```python
from build123d import *

# Parameters (mm, degrees)
BOSS_EXTRUDE1_DEPTH = 600
SKETCH2_W           = 40
SKETCH2_H           = 20
BOSS_EXTRUDE2_DEPTH = 40
FILLET1_R           = 10
SKETCH3_R           = 12
CUT_EXTRUDE1_DEPTH  = 40


with BuildPart() as part:
    # Sketch1 → Boss-Extrude1 (new body)
    with BuildSketch(Plane(origin=(0, 0, 0), x_dir=(1, 0, 0), z_dir=(0, 1, 0))):
        with BuildLine():
            Line((9.494919477, 2.658080263), (9.010919477, 2.658080263))
            ThreePointArc((9.010919477, 2.658080263), (8.651709233, 2.806870018), (8.502919477, 3.166080263))
            Line((8.502919477, 3.166080263), (8.502919477, 5.515080263))
            ThreePointArc((8.502919477, 5.515080263), (8.354129722, 5.874290508), (7.994919477, 6.023080263))
            Line((7.994919477, 6.023080263), (7.269000139, 6.023080263))
            ThreePointArc((7.269000139, 6.023080263), (7.074596955, 5.984411065), (6.909789894, 5.874290508))
            Line((6.909789894, 5.874290508), (3.806709233, 2.771209846))
            ThreePointArc((3.806709233, 2.771209846), (3.696588675, 2.606402785), (3.657919477, 2.411999602))
            Line((3.657919477, 2.411999602), (3.657919477, -2.355839076))
            ThreePointArc((3.657919477, -2.355839076), (3.696588675, -2.550242259), (3.806709233, -2.71504932))
            Line((3.806709233, -2.71504932), (6.909789894, -5.818129982))
            ThreePointArc((6.909789894, -5.818129982), (7.074596955, -5.92825054), (7.269000139, -5.966919737))
            Line((7.269000139, -5.966919737), (7.994919477, -5.966919737))
            ThreePointArc((7.994919477, -5.966919737), (8.354129722, -5.818129982), (8.502919477, -5.458919737))
            Line((8.502919477, -5.458919737), (8.502919477, -3.109919737))
            ThreePointArc((8.502919477, -3.109919737), (8.651709233, -2.750709492), (9.010919477, -2.601919737))
            Line((9.010919477, -2.601919737), (9.494919477, -2.601919737))
            ThreePointArc((9.494919477, -2.601919737), (9.854129722, -2.750709492), (10.002919477, -3.109919737))
            Line((10.002919477, -3.109919737), (10.002919477, -8.471919737))
            ThreePointArc((10.002919477, -8.471919737), (9.563579649, -9.532579909), (8.502919477, -9.971919737))
            Line((8.502919477, -9.971919737), (3.140919477, -9.971919737))
            ThreePointArc((3.140919477, -9.971919737), (2.781709233, -9.823129982), (2.632919477, -9.463919737))
            Line((2.632919477, -9.463919737), (2.632919477, -8.979919737))
            ThreePointArc((2.632919477, -8.979919737), (2.781709233, -8.620709492), (3.140919477, -8.471919737))
            Line((3.140919477, -8.471919737), (5.489919477, -8.471919737))
            ThreePointArc((5.489919477, -8.471919737), (5.849129722, -8.323129982), (5.997919477, -7.963919737))
            Line((5.997919477, -7.963919737), (5.997919477, -7.238000398))
            ThreePointArc((5.997919477, -7.238000398), (5.95925028, -7.043597215), (5.849129722, -6.878790154))
            Line((5.849129722, -6.878790154), (2.746049061, -3.775709492))
            ThreePointArc((2.746049061, -3.775709492), (2.581242, -3.665588935), (2.386838816, -3.626919737))
            Line((2.386838816, -3.626919737), (-2.380999861, -3.626919737))
            ThreePointArc((-2.380999861, -3.626919737), (-2.575403045, -3.665588935), (-2.740210106, -3.775709492))
            Line((-2.740210106, -3.775709492), (-5.843290767, -6.878790154))
            ThreePointArc((-5.843290767, -6.878790154), (-5.953411325, -7.043597215), (-5.992080523, -7.238000398))
            Line((-5.992080523, -7.238000398), (-5.992080523, -7.963919737))
            ThreePointArc((-5.992080523, -7.963919737), (-5.843290767, -8.323129982), (-5.484080523, -8.471919737))
            Line((-5.484080523, -8.471919737), (-3.135080523, -8.471919737))
            ThreePointArc((-3.135080523, -8.471919737), (-2.775870278, -8.620709492), (-2.627080523, -8.979919737))
            Line((-2.627080523, -8.979919737), (-2.627080523, -9.463919737))
            ThreePointArc((-2.627080523, -9.463919737), (-2.775870278, -9.823129982), (-3.135080523, -9.971919737))
            Line((-3.135080523, -9.971919737), (-8.497080523, -9.971919737))
            ThreePointArc((-8.497080523, -9.971919737), (-9.557740694, -9.532579909), (-9.997080523, -8.471919737))
            Line((-9.997080523, -8.471919737), (-9.997080523, -3.109919737))
            ThreePointArc((-9.997080523, -3.109919737), (-9.848290767, -2.750709492), (-9.489080523, -2.601919737))
            Line((-9.489080523, -2.601919737), (-9.005080523, -2.601919737))
            ThreePointArc((-9.005080523, -2.601919737), (-8.645870278, -2.750709492), (-8.497080523, -3.109919737))
            Line((-8.497080523, -3.109919737), (-8.497080523, -5.458919737))
            ThreePointArc((-8.497080523, -5.458919737), (-8.348290767, -5.818129982), (-7.989080523, -5.966919737))
            Line((-7.989080523, -5.966919737), (-7.263161184, -5.966919737))
            ThreePointArc((-7.263161184, -5.966919737), (-7.068758, -5.92825054), (-6.903950939, -5.818129982))
            Line((-6.903950939, -5.818129982), (-3.800870278, -2.71504932))
            ThreePointArc((-3.800870278, -2.71504932), (-3.69074972, -2.550242259), (-3.652080523, -2.355839076))
            Line((-3.652080523, -2.355839076), (-3.652080523, 2.411999602))
            ThreePointArc((-3.652080523, 2.411999602), (-3.69074972, 2.606402785), (-3.800870278, 2.771209846))
            Line((-3.800870278, 2.771209846), (-6.903950939, 5.874290508))
            ThreePointArc((-6.903950939, 5.874290508), (-7.068758, 5.984411065), (-7.263161184, 6.023080263))
            Line((-7.263161184, 6.023080263), (-7.989080523, 6.023080263))
            ThreePointArc((-7.989080523, 6.023080263), (-8.348290767, 5.874290508), (-8.497080523, 5.515080263))
            Line((-8.497080523, 5.515080263), (-8.497080523, 3.166080263))
            ThreePointArc((-8.497080523, 3.166080263), (-8.645870278, 2.806870018), (-9.005080523, 2.658080263))
            Line((-9.005080523, 2.658080263), (-9.489080523, 2.658080263))
            ThreePointArc((-9.489080523, 2.658080263), (-9.848290767, 2.806870018), (-9.997080523, 3.166080263))
            Line((-9.997080523, 3.166080263), (-9.997080523, 8.528080263))
            ThreePointArc((-9.997080523, 8.528080263), (-9.557740694, 9.588740435), (-8.497080523, 10.028080263))
            Line((-8.497080523, 10.028080263), (-3.135080523, 10.028080263))
            ThreePointArc((-3.135080523, 10.028080263), (-2.775870278, 9.879290508), (-2.627080523, 9.520080263))
            Line((-2.627080523, 9.520080263), (-2.627080523, 9.036080263))
            ThreePointArc((-2.627080523, 9.036080263), (-2.775870278, 8.676870018), (-3.135080523, 8.528080263))
            Line((-3.135080523, 8.528080263), (-5.484080523, 8.528080263))
            ThreePointArc((-5.484080523, 8.528080263), (-5.843290767, 8.379290508), (-5.992080523, 8.020080263))
            Line((-5.992080523, 8.020080263), (-5.992080523, 7.294160924))
            ThreePointArc((-5.992080523, 7.294160924), (-5.953411325, 7.099757741), (-5.843290767, 6.93495068))
            Line((-5.843290767, 6.93495068), (-2.740210106, 3.831870018))
            ThreePointArc((-2.740210106, 3.831870018), (-2.575403045, 3.72174946), (-2.380999861, 3.683080263))
            Line((-2.380999861, 3.683080263), (2.386838816, 3.683080263))
            ThreePointArc((2.386838816, 3.683080263), (2.581242, 3.72174946), (2.746049061, 3.831870018))
            Line((2.746049061, 3.831870018), (5.849129722, 6.93495068))
            ThreePointArc((5.849129722, 6.93495068), (5.95925028, 7.099757741), (5.997919477, 7.294160924))
            Line((5.997919477, 7.294160924), (5.997919477, 8.020080263))
            ThreePointArc((5.997919477, 8.020080263), (5.849129722, 8.379290508), (5.489919477, 8.528080263))
            Line((5.489919477, 8.528080263), (3.140919477, 8.528080263))
            ThreePointArc((3.140919477, 8.528080263), (2.781709233, 8.676870018), (2.632919477, 9.036080263))
            Line((2.632919477, 9.036080263), (2.632919477, 9.520080263))
            ThreePointArc((2.632919477, 9.520080263), (2.781709233, 9.879290508), (3.140919477, 10.028080263))
            Line((3.140919477, 10.028080263), (8.502919477, 10.028080263))
            ThreePointArc((8.502919477, 10.028080263), (9.563579649, 9.588740435), (10.002919477, 8.528080263))
            Line((10.002919477, 8.528080263), (10.002919477, 3.166080263))
            ThreePointArc((10.002919477, 3.166080263), (9.854129722, 2.806870018), (9.494919477, 2.658080263))
        make_face()
        with BuildLine():
            Line((2.127820321, -2.276425703), (2.307425444, -2.096820581))
            ThreePointArc((2.307425444, -2.096820581), (2.508857494, -1.328387548), (1.938052984, -0.775896455))
            ThreePointArc((1.938052984, -0.775896455), (2.098419477, 0.028080263), (1.938052984, 0.832056981))
            ThreePointArc((1.938052984, 0.832056981), (2.508857494, 1.384548074), (2.307425444, 2.152981107))
            Line((2.307425444, 2.152981107), (2.127820321, 2.332586229))
            ThreePointArc((2.127820321, 2.332586229), (1.359387288, 2.53401828), (0.806896195, 1.963213769))
            ThreePointArc((0.806896195, 1.963213769), (0.002919477, 2.123580263), (-0.801057241, 1.963213769))
            ThreePointArc((-0.801057241, 1.963213769), (-1.353548333, 2.53401828), (-2.121981366, 2.332586229))
            Line((-2.121981366, 2.332586229), (-2.301586489, 2.152981107))
            ThreePointArc((-2.301586489, 2.152981107), (-2.503018539, 1.384548074), (-1.932214029, 0.832056981))
            ThreePointArc((-1.932214029, 0.832056981), (-2.092580523, 0.028080263), (-1.932214029, -0.775896455))
            ThreePointArc((-1.932214029, -0.775896455), (-2.503018539, -1.328387548), (-2.301586489, -2.096820581))
            Line((-2.301586489, -2.096820581), (-2.121981366, -2.276425703))
            ThreePointArc((-2.121981366, -2.276425703), (-1.353548333, -2.477857754), (-0.801057241, -1.907053243))
            ThreePointArc((-0.801057241, -1.907053243), (0.002919477, -2.067419737), (0.806896195, -1.907053243))
            ThreePointArc((0.806896195, -1.907053243), (1.359387288, -2.477857754), (2.127820321, -2.276425703))
        make_face(mode=Mode.SUBTRACT)
    extrude(amount=BOSS_EXTRUDE1_DEPTH)

    # Sketch2 → Boss-Extrude2 (add)
    with BuildSketch(Plane(origin=(0, 600, 0), x_dir=(1, 0, 0), z_dir=(0, 1, 0))):
        Rectangle(SKETCH2_W, SKETCH2_H)
    extrude(amount=BOSS_EXTRUDE2_DEPTH)

    # Fillet1
    fillet1_edges = [part.edges().sort_by_distance(p)[0] for p in [
        (20, 640, 0),
        (-20, 640, 0),
    ]]
    fillet(fillet1_edges, radius=FILLET1_R)

    # Sketch3 → Cut-Extrude1 (cut)
    with BuildSketch(Plane.XY.offset(10)):
        with Locations((0, 620)):
            Circle(SKETCH3_R)
    extrude(amount=-CUT_EXTRUDE1_DEPTH, mode=Mode.SUBTRACT)


solid = part.part
```
Read the model definition and answer for the solid it produces. Units are mm, in the model's axes. A direction names the side the tool comes from. Round coordinates to 2 decimals unless told otherwise and drop trailing zeros. Write each loop counter-clockwise with the first axis right and the second up, starting at its lowest first coordinate (ties: lowest second). Pieces come first, ordered by that corner, then holes. Notation, with made-up numbers: (21, -1.75) - (33, -1.75) arc R16 ccw to (33, 14.25) - close; hole circle Ø7 at (66, 59). An arc over 180 degrees is marked (long way). Use CSV: the item, a comma, the result in double quotes.
Q1. Each of these flat-tipped pins is pushed along its axis until it touches: pin 1 Ø3 at (y, z) = (477, -3.5) entering from +X; pin 2 Ø2.5 at (y, z) = (151, 0) entering from -X; pin 3 Ø1.6 at (x, y) = (-7, 320.5) entering from +Z. Where does it stop, or does it pass through?
Values:
pin 1,"stops at x = 10"
pin 2,"stops at x = -3.65"
pin 3,"stops at z = 9.97"
Q2. Find section A-A, the plane y = 620. Write down the section's boundary in (x, z), then the cut area to 3 significant figures.
Values:
outline,"(-20, -10) - (-12, -10) - (-12, 10) - (-20, 10) - close; (12, -10) - (20, -10) - (20, 10) - (12, 10) - close"
area,"320 mm²"
Q3. Straight lines are drawn through the part: line 1 along X through (y, z) = (235, -1.25); line 2 along X through (y, z) = (158, 8); line 3 along Y through (x, z) = (0, 0.75). For each, find the intervals that lie inside material, in ascending order.
Values:
line 1,"x = -3.65 to -2.45, 2.46 to 3.66"
line 2,"x = -10 to -5.99, 6 to 10"
line 3,"y = 600 to 608, 632 to 640"
Q4. A tool of negligible diameter and unlimited length cuts with its end or side. For faces 5 (the flat face through (0, 600, 4)), 6 (the cylindrical face through (-17.15, 636.99, -0.14)), from which of +Z, -Z, +X, -X, +Y, -Y can it reach the whole face along a straight path? Write none if from no direction.
Values:
face 5,"-Y"
face 6,"+Z, -Z, -X, +Y"
Q5. Determine the mould class of faces 1 (the flat face through (20, 615, 0)), 2 (the flat face through (0, 640, 0)), 3 (the cylindrical face through (6.45, 630.12, 0.14)), 4 (the flat face through (-20, 615, 0)) for opening direction X: +X half, -X half, draft (parallel to the pull), parting line (faces both ways), or undercut.
Values:
face 1,"+X half"
face 2,"draft"
face 3,"undercut"
face 4,"-X half"
